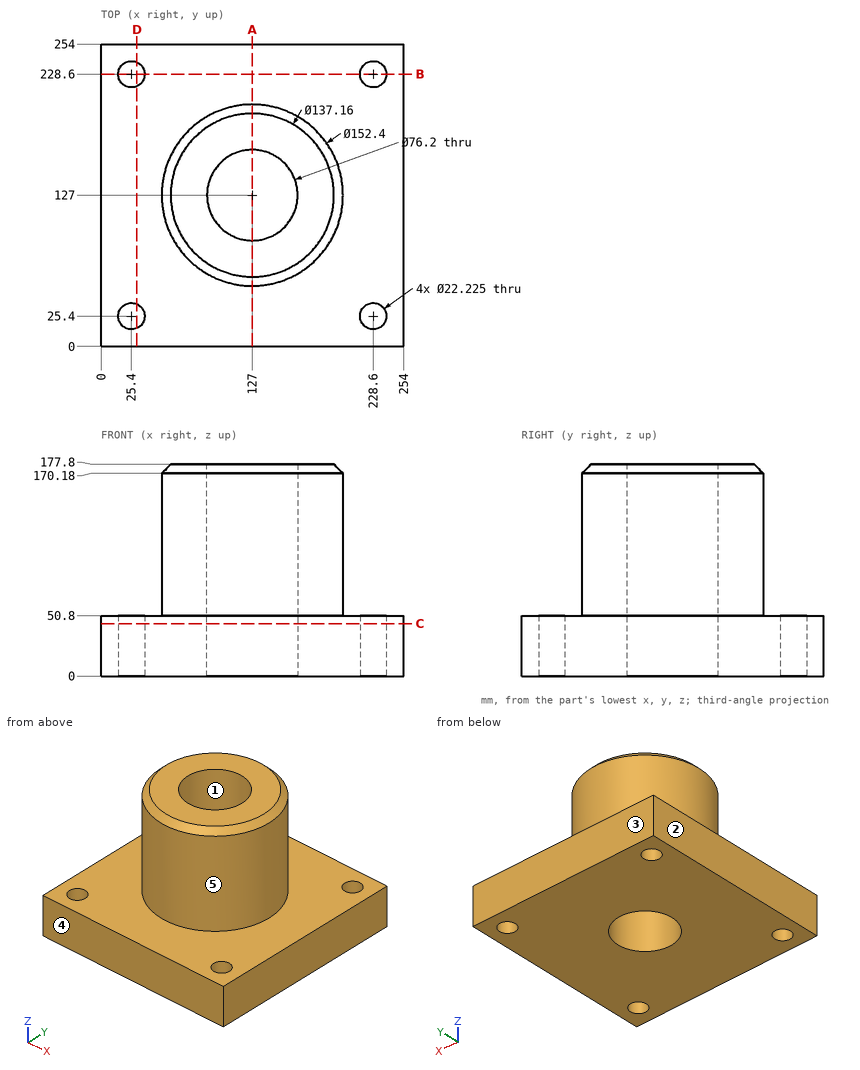
Print and shaded views of the part. All mm, measured from the part's lowest x, y and z. A direction names the side the tool comes from. Give positions to 0.01 mm unless a question says otherwise; leave off trailing zeros. Write each loop counter-clockwise with the first axis right and the second up, starting at its lowest first coordinate (ties: lowest second). Pieces come first, ordered by that corner, then holes. Notation, with made-up numbers: M 6,-29.5 L 15,-29.5 A10 cw 15,-14.5 Z; hole C 53.25,30 d4. An arc over 180 degrees is marked long. Use a Markdown table: item, result.
1) Cut at D-D (x = 30). List the corners of the cut face in (y, z), and give its area (3 significant figures).
Responses:
| item | result |
|---|---|
| outline | M 0,0 L 15.28,0 L 15.28,50.8 L 0,50.8 Z; M 35.52,0 L 218.48,0 L 218.48,50.8 L 35.52,50.8 Z; M 238.72,0 L 254,0 L 254,50.8 L 238.72,50.8 Z |
| area | 10,800 mm2 |
2) Cut at B-B (y = 228.6). List the corners of the cut face in (x, z).
Responses:
| item | result |
|---|---|
| outline | M 0,0 L 14.29,0 L 14.29,50.8 L 0,50.8 Z; M 36.51,0 L 217.49,0 L 217.49,50.8 L 36.51,50.8 Z; M 239.71,0 L 254,0 L 254,50.8 L 239.71,50.8 Z |
3) Pull direction Y, two halves, no side cores. Call the marked faces 1, 2 and 3: +Y half, -Y half, draft (parallel to the pull), parting line (faces both ways), or undercut.
Responses:
| item | result |
|---|---|
| face 1 | undercut |
| face 2 | draft |
| face 3 | +Y half |
4) Cut at C-C (z = 44). List the corners of the cut face in (x, y) (1 decimal), and give its area (3 significant figures).
Responses:
| item | result |
|---|---|
| outline | M 0,0 L 254,0 L 254,254 L 0,254 Z; hole C 25.4,25.4 d22.2; hole C 25.4,228.6 d22.2; hole C 127,127 d76.2; hole C 228.6,25.4 d22.2; hole C 228.6,228.6 d22.2 |
| area | 58,400 mm2 |
5) Pin check, flat tips, straight feed: pin 1 (8 mm diameter, centred on x = 141.5, z = 115, fed in from -Y); pin 2 (10 mm diameter, centred on y = 66.5, z = 153.5, fed in from -X); pin 3 (1.5 mm diameter, centred on y = 118.5, z = 90, fed in from -X); pin 4 (18 mm diameter, centred on x = 25.4, y = 25.4, fed in from +Z). Stop position of each tip, or through.
Responses:
| item | result |
|---|---|
| pin 1 | stops at y = 51.53 |
| pin 2 | stops at x = 74.79 |
| pin 3 | stops at x = 51.2 |
| pin 4 | passes through |
6) Drill centre lines: line 1 (Y direction, x = 228.6, z = 10); line 2 (X direction, y = 228, z = 31); line 3 (Y direction, x = 127, z = 87). Where is each one in solid material? Low to high. Write a range as from..to.
Responses:
| item | result |
|---|---|
| line 1 | y = 0..14.29, 36.51..217.49, 239.71..254 |
| line 2 | x = 0..14.3, 36.5..217.5, 239.7..254 |
| line 3 | y = 50.8..88.9, 165.1..203.2 |
7) Tool access for the marked faces 4 and 5: list every direction of +Z, -Z, +X, -X, +Y, -Y with a clear straight run to the whole face (end or side of a thin tool).
Responses:
| item | result |
|---|---|
| face 4 | +Z, -Z, +X, -X, -Y |
| face 5 | +Z |
8) Cut at A-A (x = 127). List the corners of the cut face in (y, z), and give its area (3 significant figures).
Responses:
| item | result |
|---|---|
| outline | M 0,0 L 88.9,0 L 88.9,177.8 L 58.42,177.8 L 50.8,170.18 L 50.8,50.8 L 0,50.8 Z; M 165.1,0 L 254,0 L 254,50.8 L 203.2,50.8 L 203.2,170.18 L 195.58,177.8 L 165.1,177.8 Z |
| area | 18,700 mm2 |
